Autodesk Inventor part; units mm, degrees
ref_plane "YZ Plane" through (0, 0, 0) normal (1, 0, 0) x (0, 1, 0)
ref_plane "XZ Plane" through (0, 0, 0) normal (0, 1, 0) x (-1, 0, 0)
ref_plane "XY Plane" through (0, 0, 0) normal (0, 0, 1) x (1, 0, 0)
sketch "Sketch1" plane through (0, 0, 0) normal (0, 0, 1) x (1, 0, 0)
  line L0 (0, 0) -> (-20, 0)
  line L1 (-20, 0) -> (-20, 48)
  line L2 (-20, 48) -> (0, 48)
  line L3 (0, 48) -> (0, 0)
  line L4 (-20, 0) -> (21, 0)
  line L5 (21, 0) -> (21, -20)
  line L6 (21, -20) -> (-20, -20)
  line L7 (-20, -20) -> (-20, 0)
  line L8 (21, -11.45) -> (-2.55, -11.45)
  line L9 (-2.55, -11.45) -> (-2.55, -8.55)
  line L10 (-2.55, -8.55) -> (21, -8.55)
  line L11 (21, -8.55) -> (21, -11.45)
  line L12 (-2.55, -11.45) -> (-5.45, -11.45)
  line L13 (-5.45, -11.45) -> (-5.45, 41.45)
  line L14 (-5.45, 41.45) -> (-2.55, 41.45)
  line L15 (-2.55, 41.45) -> (-2.55, -11.45)
  line L16 (-2.55, 41.45) -> (-2.55, 38.55)
  line L17 (0, 38.55) -> (0, 41.45)
  line L18 (-12.95, 0) -> (-7.05, 0)
  line L19 (-7.05, 0) -> (-7.05, 25)
  line L20 (-7.05, 25) -> (-12.95, 25)
  line L21 (-12.95, 25) -> (-12.95, 0)
  point P0 (21, -10)
  point P1 (-2.5, 40)
  point P2 (-4, 13.49)
  point P3 (-10, 0)
  point P4 (-10, 48)
  dimension "d0" = 20
  dimension "d1" = 48
  dimension "d2" = 41
  dimension "d3" = 20
  dimension "d5" = 1.45
  dimension "d6" = 2.9
  dimension "d7" = 2.9
  dimension "d8" = 8
  dimension "d11" = 4
  dimension "d12" = 1.45
  dimension "d13" = 1.45
  dimension "d14" = 1.45
  dimension "d16" = 2.95
  dimension "d17" = 5.9
  dimension "d18" = 25
extrude "Extrusion1" add sketch "Sketch1" along normal blind 1
extrude "Extrusion2" add sketch "Sketch1" against normal blind 7 contours L13 L14 L15 L0 | L0 L15 L9 L12 L13 | L10 L5 L8 L9
extrude "Extrusion3" add sketch "Sketch1" against normal blind 3 contours L0 L21 L20 L19
equation "\"d7\" = d6"
equation "\"d10\" = d6"
properties part number "cache_nappe_cote"
Build history of the part. All positions in model axes, mm. A direction names the side the tool comes from. Coordinates: 2 decimals unless noted, no trailing zeros. Write each loop counter-clockwise with the first axis right and the second up, starting at its lowest first coordinate (ties: lowest second). Pieces come first, ordered by that corner, then holes.
(1) Cut at A-A on z = -1.75. List the corners of the cut face in (x, y), and give its area (3 significant figures).
(2) Cut at B-B on y = 8.5. List the corners of the cut face in (x, z).
(3) 3-axis set-ups, long thin cutter, end or side, ignore diameter. For faces 1 (the flat face through (-7.05, 12, -1)), 2 (the flat face through (-12.95, 13, -1)), 3 (the flat face through (8, -11.45, -3)), 4 (the flat face through (9, -8.55, -3)): which of +Z, -Z, +X, -X, +Y, -Y reach the whole face in a straight line?
(4) Pin check, flat tips, straight feed: pin 1 Ø0.8 at (x, z) = (8.5, 0.5) entering from +Y; pin 2 Ø3.5 at (x, z) = (5.5, -4) entering from -Y; pin 3 Ø0.9 at (x, z) = (-9, -2) entering from -Y. Stop position of each tip, or through.
(5) Mould opens along X. For faces 5 (the flat face through (-5.45, 15, -3)), 6 (the flat face through (-2.55, 17, -3)), 7 (the flat face through (-4, 7, 1)) say: pulls with the +X half, pulls with the -X half, needs draft (parallel to the pull), parting line crosses it, or undercut.
(6) Cut at C-C on x = 17. List the corners of the cut face in (y, z), and give its area (3 significant figures).
(7) Cut at D-D on z = -5.5. List the corners of the cut face in (x, y).
(8) Drill centre lines: line 1 (X direction, y = 24.5, z = -2.5); line 2 (X direction, y = 29, z = -4.5); line 3 (Y direction, x = 6.5, z = -3.25). Where is each one in solid material? Low to high.
Working result:
1. outline: (-12.95, 0) - (-7.05, 0) - (-7.05, 25) - (-12.95, 25) - close; (-5.45, -11.45) - (21, -11.45) - (21, -8.55) - (-2.55, -8.55) - (-2.55, 41.45) - (-5.45, 41.45) - close
1. area: 369 mm2
2. outline: (-20, 0) - (-12.95, 0) - (-12.95, -3) - (-7.05, -3) - (-7.05, 0) - (-5.45, 0) - (-5.45, -7) - (-2.55, -7) - (-2.55, 0) - (0, 0) - (0, 1) - (-20, 1) - close
3. face 1: -Z, +Y, -Y
3. face 2: -Z, -X, +Y, -Y
3. face 3: -Z, +X, -X, -Y
3. face 4: -Z, +X, +Y
4. pin 1: stops at y = 0
4. pin 2: stops at y = -11.45
4. pin 3: stops at y = 0
5. face 5: undercut
5. face 6: pulls with the +X half
5. face 7: needs draft
6. outline: (-20, 0) - (-11.45, 0) - (-11.45, -7) - (-8.55, -7) - (-8.55, 0) - (0, 0) - (0, 1) - (-20, 1) - close
6. area: 40.3 mm2
7. outline: (-5.45, -11.45) - (21, -11.45) - (21, -8.55) - (-2.55, -8.55) - (-2.55, 41.45) - (-5.45, 41.45) - close
8. line 1: x = -12.95 to -7.05, -5.45 to -2.55
8. line 2: x = -5.45 to -2.55
8. line 3: y = -11.45 to -8.55
